Part print with two shaded views. Sizes in mm from the minimum x, y, z corner. A direction names the side the tool comes from. Round coordinates to 2 decimals unless told otherwise and drop trailing zeros. Write each loop counter-clockwise with the first axis right and the second up, starting at its lowest first coordinate (ties: lowest second). Pieces come first, ordered by that corner, then holes.
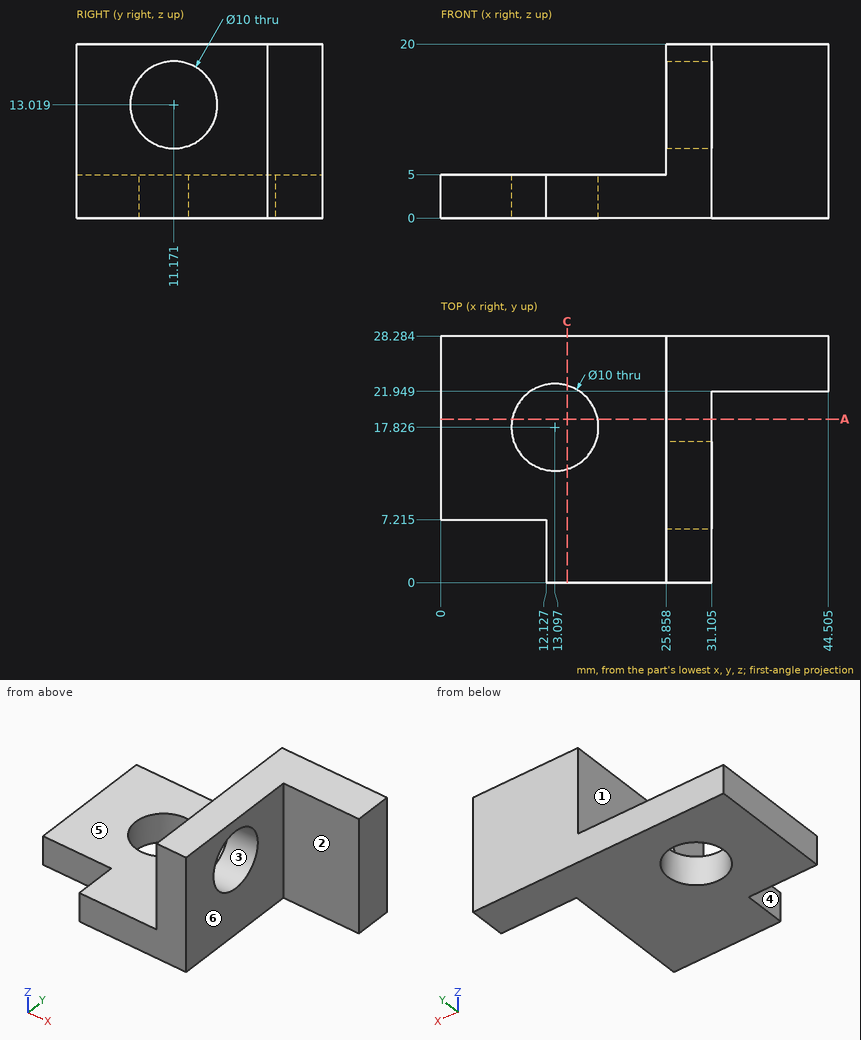
Q1. Wall check: L1, parallel to Z at x = 28, y = 11.25; L2, parallel to X at y = 26.25, z = 13.25 (1 decimal); L3, parallel to Y at x = 38, z = 5. Give the ranges that are in metal, low to high.
Values follow:
L1: z = 0 to 8.02, 18.02 to 20
L2: x = 25.9 to 44.5
L3: y = 21.95 to 28.28
Q2. Mould opens along Y. For the marked faces 1, 2 and 3 say: +Y half, -Y half, draft (parallel to the pull), parting line (faces both ways), or undercut.
Values follow:
face 1: draft
face 2: -Y half
face 3: undercut
Q3. Which spindle directions (+Z, -Z, +X, -X, +Y, -Y) get a long thin tool onto all of the face, cutting with end or side? Do the marked faces 4, 5 and 6. Say none if no direction does.
Values follow:
face 4: +Z, -Z, -X, -Y
face 5: +Z, -X, +Y, -Y
face 6: +Z, -Z, +X, -Y
Q4. Cut at A-A on y = 18.75. Write the cut outline in (x, z) (1 decimal).
Values follow:
outline: (0, 0) - (8.2, 0) - (8.2, 5) - (0, 5) - close; (18, 0) - (31.1, 0) - (31.1, 20) - (25.9, 20) - (25.9, 5) - (18, 5) - close
Q5. Drop flat-ended pins along their axis: pin 1 (3 mm diameter, centred on y = 11, z = 8, fed in from -X); pin 2 (1.5 mm diameter, centred on x = 28.5, y = 14.5, fed in from -Z); pin 3 (13 mm diameter, centred on x = 10, y = 15, fed in from +Z); pin 4 (4 mm diameter, centred on y = 3, z = 2, fed in from -X). Give the stop position or say it passes through.
Values follow:
pin 1: stops at x = 25.86
pin 2: stops at z = 0
pin 3: stops at z = 5
pin 4: stops at x = 12.13
Q6. Cut at C-C on x = 14.5. Write the cut outline in (y, z) (1 decimal).
Values follow:
outline: (0, 0) - (13, 0) - (13, 5) - (0, 5) - close; (22.6, 0) - (28.3, 0) - (28.3, 5) - (22.6, 5) - close
